For this review, take the finished solid that the model builds, in its own axes (mm). Face numbers are marked on the shaded views. A direction names the side the tool comes from. Coordinates: 2 decimals unless noted, no trailing zeros. Loops run counter-clockwise (first coordinate to the right, second up) from the corner with the lowest first, then second, coordinate; pieces in that order, holes last. Notation, with made-up numbers: (2, 40) - (37, 40) arc R19 cw to (37, 49) - close; hole circle Ø2 at (8, 49.5). An arc over 180 degrees is marked (long way). Use one line per item in the form item = value. Start each with the question number.
1. Add section D-D on z = 25. Give the boundary of the cut face in (x, y), and give its area (3 significant figures).
2. For pin 1 Ø18 at (x, z) = (-42.5, -35) entering from +Y; pin 2 Ø5 at (x, y) = (31.5, 25) entering from -Z; pin 3 Ø22 at (x, z) = (32.5, 22) entering from -Y; pin 4 Ø4 at (x, y) = (0, 84) entering from -Z, all flat-tipped, find the tip position at first contact; note any pin that passes through.
3. Draft analysis for pull direction Z (two halves, no side actions). For the marked faces 1, 2 and 3, state which applies: +Z half, -Z half, draft (parallel to the pull), parting line (faces both ways), or undercut.
4. Add section B-B on y = 8. Give the boundary of the cut face in (x, z), and give its area (3 significant figures).
5. Add section C-C on x = -42.5. Give the boundary of the cut face in (y, z), and give its area (4 significant figures).
6. Add section A-A on x = 19. Give the boundary of the cut face in (y, z).
7. To check wall thickness, follow probe 1 along Z at (x, y) = (-42.5, 94.25); probe 2 along Y at (x, z) = (15, 28); probe 3 along X at (y, z) = (91, -35). State the ranges of each line that lie inside material, in increasing order.
8. Machinability: for the marked faces 4, 5 and 6, which of the approach directions +Z, -Z, +X, -X, +Y, -Y give a long, thin tool a straight path to every point of the face, cutting with its end or side? Answer none if there is none.
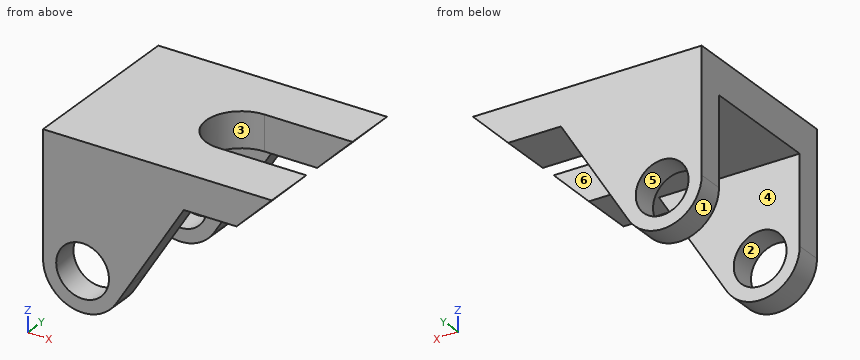
```python
from build123d import *

# Parameters (mm, degrees)
BOSS_EXTRUDE1_DEPTH     = 100
SKETCH2_W               = 30
SKETCH2_H               = 15
CUT_EXTRUDE1_DEPTH      = 73.5
SKETCH2_3_W             = 30
SKETCH2_3_H             = 40
SKETCH2_3_W_2           = 61.993822349
CUT_EXTRUDE3_DEPTH      = 73.5
CUT_EXTRUDE3_DEPTH_BACK = 21


with BuildPart() as part:
    # Sketch1 → Boss-Extrude1 (new body)
    with BuildSketch(Plane(origin=(0, 0, 0), x_dir=(1, 0, 0), z_dir=(0, 1, 0))):
        with BuildLine():
            Line((15, -15), (-16.021323509, 35))
            Line((-16.021323509, 35), (-20, 35))
            ThreePointArc((-20, 35), (-42.5, 12.5), (-65, 35))
            Line((-65, 35), (-65, -35))
            Line((-65, -35), (65, -35))
            Line((65, -35), (45, -15))
            Line((45, -15), (15, -15))
        make_face()
        with BuildLine():
            ThreePointArc((-20, 35), (-20.861711534, 41.16720944), (-23.38084198, 46.862031723))
            ThreePointArc((-23.38084198, 46.862031723), (-48.66720944, 56.638288466), (-65, 35))
            Line((-65, 35), (-57.5, 35))
            ThreePointArc((-57.5, 35), (-42.5, 50), (-27.5, 35))
            Line((-27.5, 35), (-20, 35))
        make_face()
        with BuildLine():
            ThreePointArc((-65, 35), (-42.5, 12.5), (-20, 35))
            Line((-20, 35), (-27.5, 35))
            ThreePointArc((-27.5, 35), (-42.5, 20), (-57.5, 35))
            Line((-57.5, 35), (-65, 35))
        make_face()
        with BuildLine():
            Line((-16.021323509, 35), (-23.38084198, 46.862031723))
            ThreePointArc((-23.38084198, 46.862031723), (-20.861711534, 41.16720944), (-20, 35))
            Line((-20, 35), (-16.021323509, 35))
        make_face()
    extrude(amount=BOSS_EXTRUDE1_DEPTH)

    # Sketch2 → Cut-Extrude1 (cut, through all)
    with BuildSketch(Plane(origin=(0, 0, 15), x_dir=(-1, 0, 0), z_dir=(0, 0, -1))):
        with Locations((-30, 77.5)):
            Rectangle(SKETCH2_W, SKETCH2_H)
        with BuildLine():
            Line((-15, 85), (-15, 70))
            ThreePointArc((-15, 70), (5, 50), (-15, 30))
            Line((-15, 30), (-15, 15))
            Line((-15, 15), (76.993822349, 15))
            Line((76.993822349, 15), (76.993822349, 85))
            Line((76.993822349, 85), (-15, 85))
        make_face()
        with Locations((-30, 22.5)):
            Rectangle(SKETCH2_W, SKETCH2_H)
    extrude(amount=CUT_EXTRUDE1_DEPTH, mode=Mode.SUBTRACT)

    # Sketch2<3> → Cut-Extrude3 (cut, two sides)
    with BuildSketch(Plane(origin=(0, 0, 15), x_dir=(-1, 0, 0), z_dir=(0, 0, -1))) as cut_extrude3_sk:
        with Locations((-30, 50)):
            Rectangle(SKETCH2_3_W, SKETCH2_3_H)
        with Locations((-75.996911175, 50)):
            Rectangle(SKETCH2_3_W_2, SKETCH2_3_H)
        with BuildLine():
            ThreePointArc((-15, 30), (5, 50), (-15, 70))
            Line((-15, 70), (-15, 30))
        make_face()
    extrude(amount=CUT_EXTRUDE3_DEPTH, mode=Mode.SUBTRACT)
    extrude(cut_extrude3_sk.sketch, amount=-CUT_EXTRUDE3_DEPTH_BACK, mode=Mode.SUBTRACT)


solid = part.part
```
Conclusion:
q1.outline = (-65, 0) - (55, 0) - (55, 30) - (15, 30) arc R20 cw to (15, 70) - (55, 70) - (55, 100) - (-65, 100) - close
q1.area = 9,770 mm^2
q2.pin_1 = through
q2.pin_2 = 15
q2.pin_3 = 0
q2.pin_4 = -11.97
q3.face_1 = -Z half
q3.face_2 = undercut
q3.face_3 = draft
q4.outline = (-65, -35) arc R22.5 ccw to (-23.38, -46.86) - (15, 15) - (45, 15) - (65, 35) - (-65, 35) - close; hole circle Ø30 at (-42.5, -35)
q4.area = 5,730 mm^2
q5.outline = (0, -57.5) - (15, -57.5) - (15, -50) - (0, -50) - close; (0, -20) - (15, -20) - (15, 15) - (85, 15) - (85, -20) - (100, -20) - (100, 35) - (0, 35) - close; (85, -57.5) - (100, -57.5) - (100, -50) - (85, -50) - close
q5.area = 3,275 mm^2
q6.outline = (0, 15) - (30, 15) - (30, 35) - (0, 35) - close; (70, 15) - (100, 15) - (100, 35) - (70, 35) - close
q7.probe_1 = -57.5 to -50, -20 to 35
q7.probe_2 = 0 to 30, 70 to 100
q7.probe_3 = -65 to -57.5, -27.5 to -16.02
q8.face_4 = -Z, +X, -X
q8.face_5 = +Y, -Y
q8.face_6 = +Z, -Z, +X
